Autodesk Inventor part; units mm, degrees
ref_plane "YZ Plane" through (0, 0, 0) normal (1, 0, 0) x (0, 1, 0)
ref_plane "XZ Plane" through (0, 0, 0) normal (0, 1, 0) x (-1, 0, 0)
ref_plane "XY Plane" through (0, 0, 0) normal (0, 0, 1) x (1, 0, 0)
sketch "Sketch1" plane through (0, 0, 0) normal (0, 0, 1) x (1, 0, 0)
  line L0 (-250, -580) -> (0, -580)
  line L1 (0, -580) -> (0, 0)
  line L2 (0, 0) -> (-250, 0)
  line L3 (-250, 0) -> (-250, -580)
  line L4 (-250, -580) -> (0, 0) construction
  line L5 (0, -580) -> (-250, 0) construction
  arc A0 (-180, -580) -> (-250, -45) centre (-349.5833, -330.109) ccw
  circle A1 centre (0, -580) radius 50
  circle A2 centre (0, 0) radius 50
  line L6 (0, -130) -> (0, -210) construction
  line L7 (-10, -130) -> (-10, -210)
  line L8 (10, -210) -> (10, -130)
  arc A3 (10, -130) -> (-10, -130) centre (0, -130) ccw
  arc A4 (-10, -210) -> (10, -210) centre (0, -210) ccw
  line L9 (0, -370) -> (0, -450) construction
  line L10 (-10, -370) -> (-10, -450)
  line L11 (10, -450) -> (10, -370)
  arc A5 (10, -370) -> (-10, -370) centre (0, -370) ccw
  arc A6 (-10, -450) -> (10, -450) centre (0, -450) ccw
  point P0 (0, -170)
  point P1 (0, -410)
  point P2 (0, -120)
  point P3 (0, -50)
  point P4 (-50, 0)
  point P5 (-50, -580)
  point P6 (0, -530)
  point P7 (0, -460)
  point P8 (0, -360)
  point P9 (0, -220)
  dimension "d22" = 580
  dimension "d23" = 250
  dimension "d24" = 302
  dimension "d25" = 45
  dimension "d26" = 180
  dimension "d28" = 100
  dimension "d29" = 20
  dimension "d30" = 80
  dimension "d31" = 170
  dimension "d32" = 170
extrude "Plate1" add sketch "Sketch1" along normal blind 2 contours A0 L3 L2 A2 L1 A3 L7 A4 A5 L10 A6 A1 L0
sketch "Sketch2" plane through (0, 0, 0) normal (0, 0, -1) x (-1, 0, 0)
  line L0 (20, -20) -> (220, -20) construction
  line L1 (220, -20) -> (220, -40) construction
  line L2 (220, -40) -> (20, -40) construction
  line L3 (20, -40) -> (20, -20) construction
  line L4 (50, 0) -> (250, 0)
  line L5 (0, -120) -> (0, -50)
  point P0 (0, 0)
  point P1 (0, -580)
  point P2 (0, 0)
  dimension "d6" = 200
  dimension "d9" = 20
  dimension "d10" = 20
  dimension "d11" = 20
mark "Mark1"
equation "\"d2\" = Thickness"
equation "\"BendReliefWidth\" = Thickness"
equation "\"BendReliefDepth\" = 0.5 * Thickness"
equation "\"CornerReliefSize\" = 4 * Thickness"
equation "\"MinimumRemnant\" = 2 * Thickness"
equation "\"TransitionRadius\" = BendRadius"
equation "\"JacobiRadiusSize\" = BendRadius"
equation "\"GapSize\" = Thickness"
properties part number "TRM 013 top main" material "AISI 304"
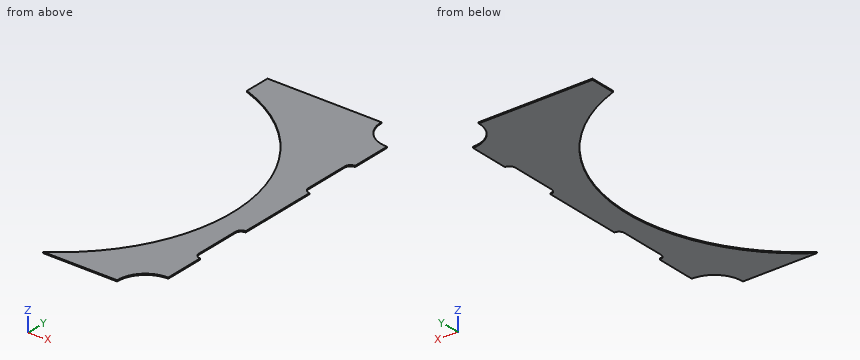
Can you work these out from the model? Positions are in its coordinate system, mm. Give positions to 0.01 mm unless a question says otherwise; leave off trailing zeros. Write each loop counter-clockwise with the first axis right and the second up, starting at its lowest first coordinate (ties: lowest second). Pieces come first, ordered by that corner, then holes. Notation, with made-up numbers: (88, 28.5) -> (116, 28.5) arc R27 ccw to (116, 65.5) -> close; hole circle Ø7 at (16, -34.75). An arc over 180 degrees is marked (long way). Write item = value, one per line.
(1) Suppose I cut it at A-A on x = -68.5. Write out the boundary of the cut face in (y, z).
Worked out:
outline = (-580, 0) -> (-440.55, 0) -> (-440.55, 2) -> (-580, 2) -> close; (-219.67, 0) -> (0, 0) -> (0, 2) -> (-219.67, 2) -> close
(2) I'm going to push a flat-ended pin straight in: P1, Ø1, axis at y = -187.5, z = 1.5, coming from the +X side. Where does the tip first touch, or does it pass through?
Worked out:
P1 = -10
(3) I need wall thicknesses on probe 1 along Y at (x, z) = (-75.5, 0.55); probe 2 along Y at (x, z) = (-104, 1.3); probe 3 along Y at (x, z) = (-191.5, 0.55). Which ranges of each line are inside material? Lowest first, please. Write a range as from..to.
Worked out:
probe_1 = -580..-456.93, -203.29..0
probe_2 = -580..-505.87, -154.35..0
probe_3 = -72.79..0
(4) Suppose I cut it at B-B on z = 1.5. Write out the boundary of the cut face in (x, y), then the cut area to 3 significant figures.
Worked out:
outline = (-250, -45) arc R302 cw to (-180, -580) -> (-50, -580) arc R50 cw to (0, -530) -> (0, -460) arc R10 cw to (-10, -450) -> (-10, -370) arc R10 cw to (0, -360) -> (0, -220) arc R10 cw to (-10, -210) -> (-10, -130) arc R10 cw to (0, -120) -> (0, -50) arc R50 cw to (-50, 0) -> (-250, 0) -> close
area = 56,300 mm^2
(5) Suppose I cut it at C-C on x = -143. Write out the boundary of the cut face in (y, z), then the cut area to 3 significant figures.
Worked out:
outline = (-580, 0) -> (-550.4, 0) -> (-550.4, 2) -> (-580, 2) -> close; (-109.82, 0) -> (0, 0) -> (0, 2) -> (-109.82, 2) -> close
area = 279 mm^2
(6) Suppose I cut it at D-D on y = -329. Write out the boundary of the cut face in (x, z), then the cut area to 3 significant figures.
Worked out:
outline = (-47.59, 0) -> (0, 0) -> (0, 2) -> (-47.59, 2) -> close
area = 95.2 mm^2
